from build123d import *

# Parameters (mm, degrees)
SKETCH_1_R          = 7.25
EXTRUDE_1_DEPTH     = 17
SKETCH_2_R          = 1.5
EXTRUDE_2_DEPTH     = 9
EXTRUDE_3_DEPTH     = 3
SKETCH_4_R          = 1
CUT_EXTRUDE_1_DEPTH = 3


with BuildPart() as part:
    # 草图1 → 凸台-拉伸1 (new body)
    with BuildSketch(Plane(origin=(0, 0, 0), x_dir=(1, 0, 0), z_dir=(0, 1, 0))):
        with Locations(Location((0, 0, 0), (0, 0, 270))):
            Circle(SKETCH_1_R)
    extrude(amount=EXTRUDE_1_DEPTH)

    # 草图2 → 凸台-拉伸2 (add)
    with BuildSketch(Plane(origin=(0, 17, 0), x_dir=(1, 0, 0), z_dir=(0, 1, 0))):
        with Locations(Location((0, 0, 0), (0, 0, 270))):
            Circle(SKETCH_2_R)
    extrude(amount=EXTRUDE_2_DEPTH)

    # 草图3 → 凸台-拉伸3 (add)
    with BuildSketch(Plane.XZ):
        with BuildLine():
            Line((-4, 7.215434845), (-4, 6.006791496))
            Line((-4, 6.006791496), (4.059674361, 6.006791496))
            Line((4.059674361, 6.006791496), (4.059674361, 7.182029245))
            ThreePointArc((4.059674361, 7.182029245), (0.034194164, 8.249929137), (-4, 7.215434845))
        make_face()
    extrude(amount=-EXTRUDE_3_DEPTH)

    # 草图4 → 切除-拉伸1 (cut)
    with BuildSketch(Plane(origin=(0, 17, 0), x_dir=(1, 0, 0), z_dir=(0, 1, 0))):
        with Locations(Location((5.5, 0, 0), (0, 0, 270))):
            Circle(SKETCH_4_R)
        with Locations(Location((-5.5, 0, 0), (0, 0, 270))):
            Circle(SKETCH_4_R)
    extrude(amount=-CUT_EXTRUDE_1_DEPTH, mode=Mode.SUBTRACT)


solid = part.part
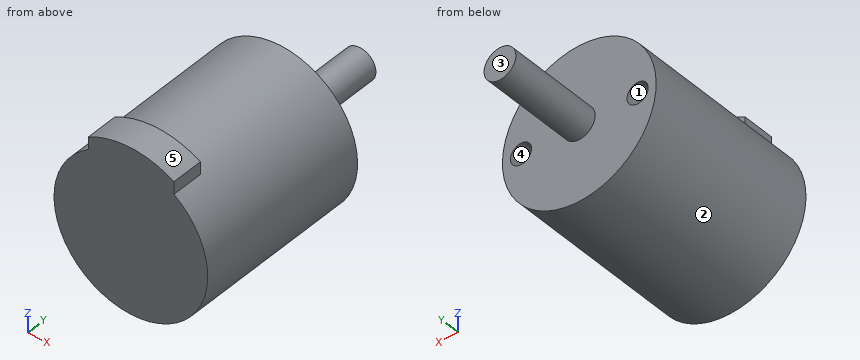
The listing builds one solid part. Answer for the finished solid, in the listing's coordinates (mm). Face numbers are marked on the shaded views. A direction names the side the tool comes from. Round coordinates to 2 decimals unless told otherwise and drop trailing zeros. Write each loop counter-clockwise with the first axis right and the second up, starting at its lowest first coordinate (ties: lowest second). Pieces come first, ordered by that corner, then holes. Notation, with made-up numbers: (-10.75, 14) - (9.25, 14) arc R20 cw to (9.25, 53) - close; hole circle Ø6 at (-1.5, 77). An arc over 180 degrees is marked (long way). Use a Markdown table: item, result. Add a question column.
1. The part is cut by section C-C (x = 0). Write down the section's boundary in (y, z).
2. Flat-ended cylindrical pins translate along their axes: P1, Ø1.8, axis at x = -5.5, z = 0, coming from the +Y side; P2, Ø2, axis at y = 22, z = 0.5, coming from the -X side; P3, Ø2.5, axis at x = -2, z = 7.5, coming from the +Y side. Find the tip coordinate at first contact, or state that the pin passes through.
3. The part is cut by section D-D (y = 20.75). Write down the section's boundary in (x, z), and give its area (3 significant figures).
4. For a pull along X with two mould halves and no side action, classify the marked faces 1, 2 and 3 as +X half, -X half, draft (parallel to the pull), parting line (faces both ways), or undercut.
5. A tool of negligible diameter and unlimited length cuts with its end or side. For the marked faces 4 and 5, from which of +Z, -Z, +X, -X, +Y, -Y can it reach the whole face along a straight path? Write none if from no direction.
6. Consider line 1 (X direction, y = 14.9, z = 0); line 2 (Y direction, x = 3.5, z = 3.5); line 3 (Z direction, x = -5, y = 15.5). Determine where each line is inside the solid, lowest interval first.
7. The part is cut by section B-B (y = 15.5). Write down the section's boundary in (x, z), and give its area (3 significant figures).
8. The part is cut by section A-A (z = 0). Write down the section's boundary in (x, y).
Reported:
| question | item | result |
|---|---|---|
| 1 | outline | (0, -7.25) - (17, -7.25) - (17, -1.5) - (26, -1.5) - (26, 1.5) - (17, 1.5) - (17, 7.25) - (3, 7.25) - (3, 8.25) - (0, 8.25) - close |
| 2 | P1 | y = 14 |
| 2 | P2 | x = -1.5 |
| 2 | P3 | y = 17 |
| 3 | outline | circle Ø3 at (0, 0) |
| 3 | area | 7.07 mm^2 |
| 4 | face 1 | undercut |
| 4 | face 2 | parting line |
| 4 | face 3 | draft |
| 5 | face 4 | +Y |
| 5 | face 5 | +Z, +Y, -Y |
| 6 | line 1 | -7.25 to -6.5, -4.5 to 4.5, 6.5 to 7.25 |
| 6 | line 2 | 0 to 17 |
| 6 | line 3 | -5.25 to -0.87, 0.87 to 5.25 |
| 7 | outline | circle Ø14.5 at (0, 0); hole circle Ø2 at (-5.5, 0); hole circle Ø2 at (5.5, 0) |
| 7 | area | 159 mm^2 |
| 8 | outline | (-7.25, 0) - (7.25, 0) - (7.25, 17) - (6.5, 17) - (6.5, 14) - (4.5, 14) - (4.5, 17) - (1.5, 17) - (1.5, 26) - (-1.5, 26) - (-1.5, 17) - (-4.5, 17) - (-4.5, 14) - (-6.5, 14) - (-6.5, 17) - (-7.25, 17) - close |
